The listing builds one solid part. Answer for the finished solid, in the listing's coordinates (mm). A direction names the side the tool comes from. Round coordinates to 2 decimals unless told otherwise and drop trailing zeros. Write each loop counter-clockwise with the first axis right and the second up, starting at its lowest first coordinate (ties: lowest second). Pieces come first, ordered by that corner, then holes. Notation, with made-up numbers: (21.5, 66) - (27.5, 66) arc R27 cw to (27.5, 88) - close; hole circle Ø7 at (-37.5, -20.75). An arc over 180 degrees is marked (long way). Return JSON: item names as keys, results as strings. Group by question number.
(1) Find the intervals of material crossed by line 1 along Y through (x, z) = (75, 3); line 2 along Y through (x, z) = (41, 10.5); line 3 along Y through (x, z) = (158, 6), in increasing order. Write a range as [from, to].
(2) Section A-A, the plane y = 112.5 is taken. Write down the section's boundary in (x, z).
(3) Each of these flat-tipped pins is pushed along its axis until it touches: pin 1 (8.5 mm diameter, centred on x = 125, y = 37.5, fed in from +Z); pin 2 (11.5 mm diameter, centred on x = 72.5, y = 38, fed in from +Z); pin 3 (4 mm diameter, centred on x = 160, y = 188.5, fed in from -Z); pin 4 (3 mm diameter, centred on x = 79, y = 190, fed in from +Z). Where does it stop, or does it pass through?
(4) Which of the six approach directions +Z, -Z, +X, -X, +Y, -Y give full straight-line access (tool end or side, diameter ignored) to faces 4 (the cylindrical face through (161.75, 191.24, 4.06)), 5 (the flat face through (78.4, 112.6, 8.8))?
(5) Determine the mould class of faces 1 (the flat face through (99, 127, 15)), 2 (the flat face through (99, 0, 7)), 3 (the flat face through (43.4, 188.6, 8)) for opening direction Y: +Y half, -Y half, draft (parallel to the pull), parting line (faces both ways), or undercut.
```python
from build123d import *

# Parameters (mm, degrees)
SKETCH_W        = 200
SKETCH_H        = 250
PAD_DEPTH       = 15
SKETCH001_R     = 3.25
POCKET_DEPTH    = 15
SKETCH002_R     = 5.2
POCKET001_DEPTH = 6.2
SKETCH003_R     = 2.5
POCKET002_DEPTH = 15
SKETCH004_R     = 3.25
POCKET003_DEPTH = 15
SKETCH005_R     = 5.2
POCKET004_DEPTH = 7


with BuildPart() as part:
    # Sketch → Pad (new body)
    with BuildSketch(Plane.XY):
        with Locations((100, 125)):
            Rectangle(SKETCH_W, SKETCH_H)
    extrude(amount=PAD_DEPTH)

    # Sketch001 (on Face6 of Pad) → Pocket (cut)
    with BuildSketch(Plane.XY.offset(15)):
        with Locations((125, 37.5)):
            Circle(SKETCH001_R)
        with Locations((75, 37.5)):
            Circle(SKETCH001_R)
        with Locations((125, 112.5)):
            Circle(SKETCH001_R)
        with Locations((75, 112.5)):
            Circle(SKETCH001_R)
    extrude(amount=-POCKET_DEPTH, mode=Mode.SUBTRACT)

    # Sketch002 (on Face5 of Pocket) → Pocket001 (cut)
    with BuildSketch(Plane.XY.offset(15)):
        with Locations((75, 112.5)):
            Circle(SKETCH002_R)
        with Locations((125, 112.5)):
            Circle(SKETCH002_R)
        with Locations((75, 37.5)):
            Circle(SKETCH002_R)
        with Locations((125, 37.5)):
            Circle(SKETCH002_R)
    extrude(amount=-POCKET001_DEPTH, mode=Mode.SUBTRACT)

    # Sketch003 (on Face5 of Pocket001) → Pocket002 (cut)
    with BuildSketch(Plane.XY.offset(15)):
        with Locations((42, 230)):
            Circle(SKETCH003_R)
        with Locations((42, 125)):
            Circle(SKETCH003_R)
        with Locations((42, 20)):
            Circle(SKETCH003_R)
        with Locations((158, 230)):
            Circle(SKETCH003_R)
        with Locations((158, 125)):
            Circle(SKETCH003_R)
        with Locations((158, 20)):
            Circle(SKETCH003_R)
    extrude(amount=-POCKET002_DEPTH, mode=Mode.SUBTRACT)

    # Sketch004 (on Face5 of Pocket002) → Pocket003 (cut)
    with BuildSketch(Plane.XY.offset(15)):
        with Locations((40, 188.5)):
            Circle(SKETCH004_R)
        with Locations((80, 188.5)):
            Circle(SKETCH004_R)
        with Locations((120, 188.5)):
            Circle(SKETCH004_R)
        with Locations((160, 188.5)):
            Circle(SKETCH004_R)
    extrude(amount=-POCKET003_DEPTH, mode=Mode.SUBTRACT)

    # Sketch005 (on Face5 of Pocket003) → Pocket004 (cut)
    with BuildSketch(Plane.XY.offset(15)):
        with Locations((40, 188.5)):
            Circle(SKETCH005_R)
        with Locations((80, 188.5)):
            Circle(SKETCH005_R)
        with Locations((120, 188.5)):
            Circle(SKETCH005_R)
        with Locations((160, 188.5)):
            Circle(SKETCH005_R)
    extrude(amount=-POCKET004_DEPTH, mode=Mode.SUBTRACT)


solid = part.part
```
Working result:
{
 "1": {"line 1": "y = [0, 34.25], [40.75, 109.25], [115.75, 250]", "line 2": "y = [0, 17.71], [22.29, 122.71], [127.29, 183.4], [193.6, 227.71], [232.29, 250]", "line 3": "y = [0, 17.5], [22.5, 122.5], [127.5, 185.94], [191.06, 227.5], [232.5, 250]"},
 "2": {"outline": "(0, 0) - (71.75, 0) - (71.75, 8.8) - (69.8, 8.8) - (69.8, 15) - (0, 15) - close; (78.25, 0) - (121.75, 0) - (121.75, 8.8) - (119.8, 8.8) - (119.8, 15) - (80.2, 15) - (80.2, 8.8) - (78.25, 8.8) - close; (128.25, 0) - (200, 0) - (200, 15) - (130.2, 15) - (130.2, 8.8) - (128.25, 8.8) - close"},
 "3": {"pin 1": "stops at z = 8.8", "pin 2": "stops at z = 15", "pin 3": "passes through", "pin 4": "stops at z = 8"},
 "4": {"face 4": "+Z, -Z", "face 5": "+Z"},
 "5": {"face 1": "draft", "face 2": "-Y half", "face 3": "undercut"}
}
